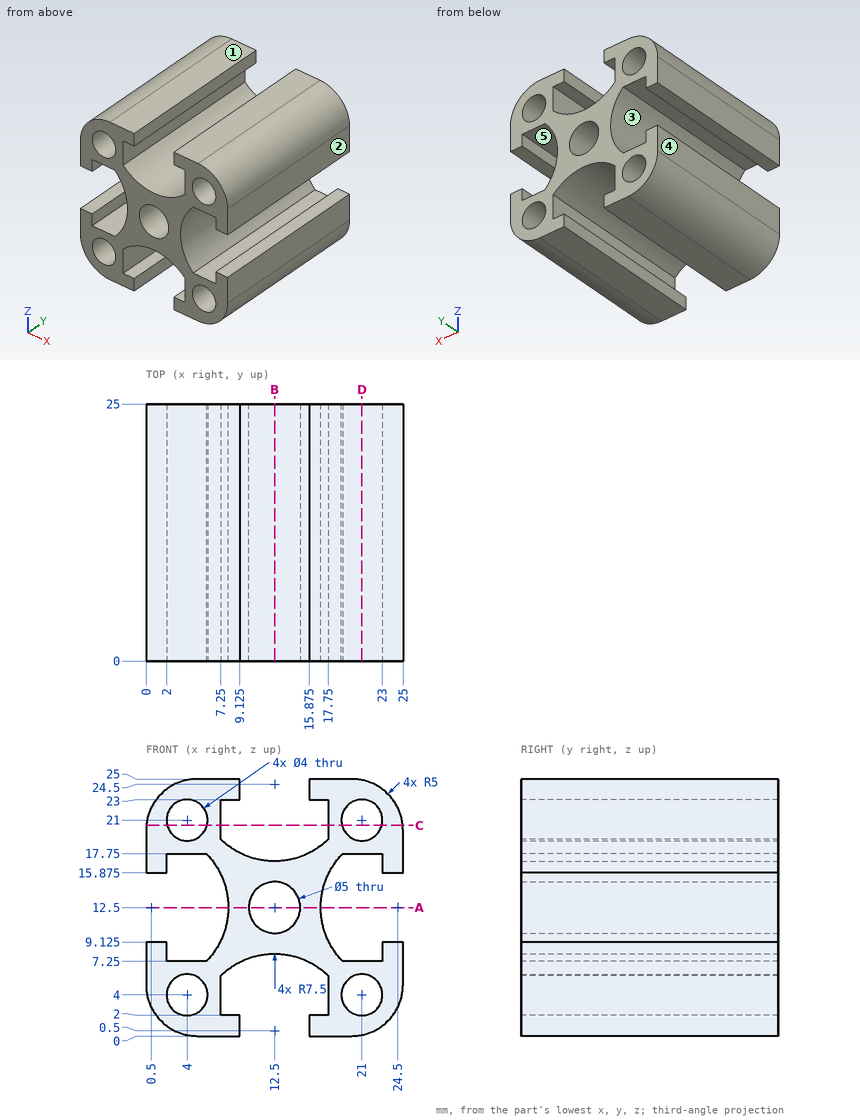
Part print with two shaded views. Sizes in mm from the minimum x, y, z corner. A direction names the side the tool comes from. Coordinates: 2 decimals unless noted, no trailing zeros. Write each loop counter-clockwise with the first axis right and the second up, starting at its lowest first coordinate (ties: lowest second). Pieces come first, ordered by that corner, then holes. Notation, with made-up numbers: (43.5, 49) - (71.5, 49) arc R18 cw to (71.5, 61) - close; hole circle Ø7 at (83.25, -33.5). An arc over 180 degrees is marked (long way). One line per item, written item: value. Start each with the question number.
1. Slice it at D-D (x = 21). Write the cut outline in (y, z), plus the area to 3 significant figures.
2. Slice it at B-B (x = 12.5). Write the cut outline in (y, z), plus the area to 3 significant figures.
3. Slice it at A-A (z = 12.5). Write the cut outline in (x, y).
4. Probe line 1 (X direction, y = 10.5, z = 1) (3 decimals); line 2 (Z direction, x = 21, y = 14.25). List the from-to ranges inside material, lowest first. Write a range as from..to.
5. Flat gauge pins, fed straight in: pin 1 (1.5 mm diameter, centred on y = 20, z = 13.5, fed in from +X); pin 2 (2 mm diameter, centred on y = 9.5, z = 0.5, fed in from -X); pin 3 (0.6 mm diameter, centred on y = 11, z = 23.5, fed in from -X); pin 4 (2.5 mm diameter, centred on x = 4, z = 4, fed in from -Y). Where does each tip first touch, or does it go through?
6. Mould opens along X. For the marked faces 1, 2 and 3 say: released by +X, released by -X, zero draft, split by the parting line, or undercut.
7. Slice it at C-C (z = 20.5). Write the cut outline in (x, y), plus the area to 3 significant figures.
8. Tool access for the marked faces 4 and 5: list every direction of +Z, -Z, +X, -X, +Y, -Y with a clear straight run to the whole face (end or side of a thin tool).
Answers below:
1. outline: (0, 0.1) - (25, 0.1) - (25, 2) - (0, 2) - close; (0, 6) - (25, 6) - (25, 7.25) - (0, 7.25) - close; (0, 17.75) - (25, 17.75) - (25, 19) - (0, 19) - close; (0, 23) - (25, 23) - (25, 24.9) - (0, 24.9) - close
1. area: 157 mm^2
2. outline: (0, 8) - (25, 8) - (25, 10) - (0, 10) - close; (0, 15) - (25, 15) - (25, 17) - (0, 17) - close
2. area: 100 mm^2
3. outline: (8, 0) - (10, 0) - (10, 25) - (8, 25) - close; (15, 0) - (17, 0) - (17, 25) - (15, 25) - close
4. line 1: x = 2..9.125, 15.875..23
4. line 2: z = 0.1..2, 6..7.25, 17.75..19, 23..24.9
5. pin 1: stops at x = 17.21
5. pin 2: stops at x = 1.43
5. pin 3: stops at x = 1.16
5. pin 4: passes through
6. face 1: zero draft
6. face 2: released by +X
6. face 3: undercut
7. outline: (0.03, 0) - (2.06, 0) - (2.06, 25) - (0.03, 25) - close; (5.94, 0) - (7.25, 0) - (7.25, 25) - (5.94, 25) - close; (17.75, 0) - (19.06, 0) - (19.06, 25) - (17.75, 25) - close; (22.94, 0) - (24.97, 0) - (24.97, 25) - (22.94, 25) - close
7. area: 168 mm^2
8. face 4: +Z, -Z, -X, +Y, -Y
8. face 5: +Y, -Y
